Verification items for the finished model (mm, model axes). Face numbers are marked on the shaded views. A direction names the side the tool comes from. Round coordinates to 2 decimals unless told otherwise and drop trailing zeros. Write each loop counter-clockwise with the first axis right and the second up, starting at its lowest first coordinate (ties: lowest second). Pieces come first, ordered by that corner, then holes.
Autodesk Inventor part; units mm, degrees
ref_plane "YZ Plane" through (0, 0, 0) normal (1, 0, 0) x (0, 1, 0)
ref_plane "XZ Plane" through (0, 0, 0) normal (0, 1, 0) x (-1, 0, 0)
ref_plane "XY Plane" through (0, 0, 0) normal (0, 0, 1) x (1, 0, 0)
sketch "Sketch1" plane through (0, 0, 0) normal (0, 0, 1) x (1, 0, 0)
  circle A0 centre (0, 0) radius 6.35
  circle A1 centre (0, 0) radius 3.175
  dimension "d0" = 12.7
  dimension "d13" = 3.175
extrude "Base" add sketch "Sketch1" along normal mid plane 25.4
sketch "Sketch4" plane through (0, 0, 12.7) normal (0, 0, 1) x (1, 0, 0)
  circle A0 centre (0, 0) radius 6.35
  circle A1 centre (0, 0) radius 4.7625
  dimension "d16" = 9.525
extrude "Extrusion4" cut sketch "Sketch4" against normal blind 1.5875
mirror "Mirror2" about plane through (0, 0, 0) normal (0, 0, 1) of "Extrusion4"
properties part number "gearbox_standoff" material "Aluminum-6061"
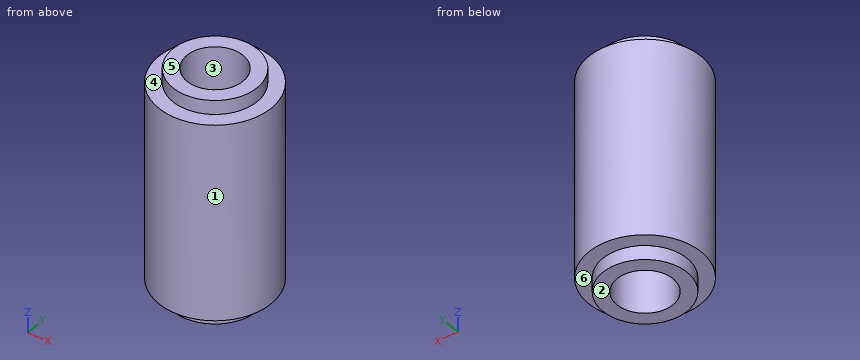
Q1. Sectioned sample at C-C (z = 5.5). Enter the section's corners in (x, y) (3 decimals), plus the area to 3 significant figures.
Recorded:
outline: circle Ø12.7 at (0, 0); hole circle Ø6.35 at (0, 0)
area: 95.0 mm2
Q2. Tool access check on the marked faces 4, 5 and 6. Record the directions out of +Z, -Z, +X, -X, +Y, -Y that give a thin tool (end or side, any length) a straight path to the whole face; none if there is none.
Recorded:
face 4: +Z
face 5: +Z, +X, -X, +Y, -Y
face 6: -Z
Q3. Sectioned sample at D-D (x = 4.5). Enter the section's corners in (y, z).
Recorded:
outline: (-4.48, -11.11) - (-1.56, -11.11) - (-1.56, -12.7) - (1.56, -12.7) - (1.56, -11.11) - (4.48, -11.11) - (4.48, 11.11) - (1.56, 11.11) - (1.56, 12.7) - (-1.56, 12.7) - (-1.56, 11.11) - (-4.48, 11.11) - close
Q4. Depth check by flat-ended pin: P1, Ø4, axis at x = -3, z = 9.5, coming from the -Y side; P2, Ø4, axis at x = 0, y = 0, coming from the -Z side; P3, Ø1, axis at y = 2, z = -4, coming from the -X side. Enter the tip coordinate at first touch or a pass-through.
Recorded:
P1: stops at y = -6.27
P2: passes through
P3: stops at x = -6.17
Q5. Material ranges on line 1 along Y through (x, z) = (0, 0.25) (3 decimals); line 2 along Z through (x, y) = (-4.5, 2.75); line 3 along Y through (x, z) = (-1.75, -1.75), recorded low to high.
Recorded:
line 1: y = -6.35 to -3.175, 3.175 to 6.35
line 2: z = -11.11 to 11.11
line 3: y = -6.1 to -2.65, 2.65 to 6.1
Q6. Release check for a two-part mould opening along Y. For the marked faces 1, 2 and 3 record: released by +Y, released by -Y, zero draft, split by the parting line, or undercut.
Recorded:
face 1: split by the parting line
face 2: zero draft
face 3: undercut
